Design review of the part built by this model. Coordinates are the model's own, in mm. A direction names the side the tool comes from. Coordinates: 2 decimals unless noted, no trailing zeros. Write each loop counter-clockwise with the first axis right and the second up, starting at its lowest first coordinate (ties: lowest second). Pieces come first, ordered by that corner, then holes. Notation, with made-up numbers: M 55.25,68.5 L 87.25,68.5 A16 cw 87.25,89.5 Z; hole C 39,32 d1. An arc over 180 degrees is marked long. Return JSON: item names as keys, results as strings. Group by question number.
```python
from build123d import *

# Parameters (mm, degrees)
CYLINDER001_R               = 4
CYLINDER001_DEPTH           = 30
CYLINDER_R                  = 2.2
CYLINDER_DEPTH              = 30
COMPOUND001_PLACEMENT_ANGLE = 60
BOX001_W                    = 114
BOX001_H                    = 52.5
BOX001_DEPTH                = 20
BOX002_W                    = 94
BOX002_H                    = 32.5
BOX002_DEPTH                = 20
BOX003_W                    = 74
BOX003_H                    = 10
BOX003_DEPTH                = 15
CYLINDER002_R               = 10
CYLINDER002_DEPTH           = 50
PAD_DEPTH                   = 4
PAD001_DEPTH                = 20
CYLINDER003_W               = 2.5
CYLINDER003_H               = 5
CYLINDER003_ANGLE           = 180
COMPOUND002_PLACEMENT_ANGLE = 60
BOX_W                       = 120
BOX_H                       = 58.5
BOX_DEPTH                   = 20
FILLET_R                    = 2


with BuildPart() as bolt_head_hole:
    # Cylinder001 → Cylinder001 (new body)
    with BuildSketch(Plane.XZ.offset(14)):
        Circle(CYLINDER001_R)
    extrude(amount=CYLINDER001_DEPTH)


with BuildPart() as bolt_hole_array_compound:
    # Cylinder → Cylinder (new body)
    with BuildSketch(Plane.XZ):
        Circle(CYLINDER_R)
    extrude(amount=CYLINDER_DEPTH)

    # Fusion002: union bolt head hole
    add(bolt_head_hole.part)


with BuildPart() as bolt_hole_array_compound_1:
    # Compound001 placement: moved
    add(bolt_hole_array_compound.part.moved(Location((-32.3149, 81.256849, 10))).rotate(Axis((-32.3149, 81.256849, 10), (0, 0, -1)), COMPOUND001_PLACEMENT_ANGLE))


with BuildPart() as part_mirroring:
    # Part__Mirroring: instance of bolt hole array compound
    add(bolt_hole_array_compound_1.part.mirror(Plane(origin=(0, 0, 0), x_dir=(0, -1, 0), z_dir=(1, 0, 0))))


with BuildPart() as obj1:
    # Box001 → Box001 (new body)
    with BuildSketch(Plane(origin=(-57, -26.25, 3), x_dir=(1, 0, 0), z_dir=(0, 0, 1))):
        with Locations((57, 26.25)):
            Rectangle(BOX001_W, BOX001_H)
    extrude(amount=BOX001_DEPTH)


with BuildPart() as obj2:
    # Box002 → Box002 (new body)
    with BuildSketch(Plane(origin=(-47, -16.25, 0), x_dir=(1, 0, 0), z_dir=(0, 0, 1))):
        with Locations((47, 16.25)):
            Rectangle(BOX002_W, BOX002_H)
    extrude(amount=BOX002_DEPTH)


with BuildPart() as switch_pocket:
    # Box003 → Box003 (new body)
    with BuildSketch(Plane(origin=(-37, -31.25, 8), x_dir=(1, 0, 0), z_dir=(0, 0, 1))):
        with Locations((37, 5)):
            Rectangle(BOX003_W, BOX003_H)
    extrude(amount=BOX003_DEPTH)


with BuildPart() as center_remove_cylinder:
    # Cylinder002 → Cylinder002 (new body)
    with BuildSketch(Plane(origin=(0, 47, -25), x_dir=(1, 0, 0), z_dir=(0, 0, 1))):
        Circle(CYLINDER002_R)
    extrude(amount=CYLINDER002_DEPTH)


with BuildPart() as extract_fusion:
    # Fusion003 base: copy of bolt hole array compound
    add(bolt_hole_array_compound_1.part)

    # Fusion003: union Part__Mirroring, obj1, obj2, switch pocket, center remove cylinder
    add(part_mirroring.part)
    add(obj1.part)
    add(obj2.part)
    add(switch_pocket.part)
    add(center_remove_cylinder.part)


with BuildPart() as bottom_body:
    # Sketch → Pad (new body)
    with BuildSketch(Plane.XY):
        with BuildLine():
            Line((-60, 29.25), (60, 29.25))
            Line((60, 29.25), (47.625, 86.066815))
            Line((32.625, 60.086053), (47.625, 86.066815))
            ThreePointArc((-32.625, 60.086053), (0, 41.25), (32.625, 60.086053))
            Line((-32.625, 60.086053), (-47.625, 86.066815))
            Line((-60, 29.25), (-47.625, 86.066815))
        make_face()
    extrude(amount=PAD_DEPTH)


with BuildPart() as bolt_wall_body:
    # Sketch001 → Pad001 (new body)
    with BuildSketch(Plane.XY):
        with BuildLine():
            Line((-47.625, 86.066815), (-32.625, 60.086053))
            ThreePointArc((-32.625, 60.086053), (0, 41.25), (32.625, 60.086053))
            Line((32.625, 60.086053), (47.625, 86.066815))
            Line((50.123562, 74.595272), (47.625, 86.066815))
            Line((44.094416, 64.152484), (50.123562, 74.595272))
            ThreePointArc((44.094416, 64.152484), (42.751879, 58.90179), (44.333925, 53.718226))
            Line((44.333925, 53.718226), (60, 29.25))
            Line((60, 29.25), (-60, 29.25))
            Line((-44.333925, 53.718226), (-60, 29.25))
            ThreePointArc((-44.333925, 53.718226), (-42.751879, 58.90179), (-44.094416, 64.152484))
            Line((-50.123562, 74.595272), (-44.094416, 64.152484))
            Line((-50.123562, 74.595272), (-47.625, 86.066815))
        make_face()
    extrude(amount=PAD001_DEPTH)


with BuildPart() as bolt_hole_array_compound001:
    # Cylinder003 → Cylinder003 (revolve)
    with BuildSketch(Plane(origin=(0, 0, 0), x_dir=(0, 0, -1), z_dir=(0, -1, 0))):
        with Locations((1.25, 2.5)):
            Rectangle(CYLINDER003_W, CYLINDER003_H)
    revolve(axis=Axis((0, 0, 0), (1, 0, 0)), revolution_arc=CYLINDER003_ANGLE)


with BuildPart() as bolt_hole_array_compound001_1:
    # Compound002 placement: moved
    add(bolt_hole_array_compound001.part.moved(Location((-39.21, 68.392051, 10))).rotate(Axis((-39.21, 68.392051, 10), (0, 0, -1)), COMPOUND002_PLACEMENT_ANGLE))


with BuildPart() as part_mirroring003:
    # Part__Mirroring003: instance of bolt hole array compound001
    add(bolt_hole_array_compound001_1.part.mirror(Plane(origin=(0, 0, 0), x_dir=(0, -1, 0), z_dir=(1, 0, 0))))


with BuildPart() as bolt_wall_body_cut:
    # Box → Box (new body)
    with BuildSketch(Plane(origin=(-60, -29.25, 0), x_dir=(1, 0, 0), z_dir=(0, 0, 1))):
        with Locations((60, 29.25)):
            Rectangle(BOX_W, BOX_H)
    extrude(amount=BOX_DEPTH)

    # Fillet
    fillet_edges = [bolt_wall_body_cut.edges().sort_by_distance(p)[0] for p in [
        (-60, -29.25, 10),
        (60, -29.25, 10),
    ]]
    fillet(fillet_edges, radius=FILLET_R)

    # Fusion: union bottom_body, bolt wall body, bolt hole array compound001, Part__Mirroring003
    add(bottom_body.part)
    add(bolt_wall_body.part)
    add(bolt_hole_array_compound001_1.part)
    add(part_mirroring003.part)

    # Cut001: cut extract fusion
    add(extract_fusion.part, mode=Mode.SUBTRACT)


solid = bolt_wall_body_cut.part
```
Item 1: The part is to be moulded in two halves that separate along X. For faces 4 (the flat face through (46.397, 68.14, 11.888)), 5 (the flat face through (40.02, 72.895, 9.86)), 6 (the flat face through (-0.8, -29.25, 7.6)), say which applies: pulls with the +X half, pulls with the -X half, needs draft (parallel to the pull), parting line crosses it, or undercut.
Item 2: Add section A-A (x = 0). Write out the cut boundary in (y, z), plus the area to 3 significant figures.
Item 3: For line 1 (X direction, y = -20, z = 17.5); line 2 (X direction, y = -9, z = 1); line 3 (Y direction, x = -4, z = 1.5), list the stretches that pass through material, from the lowest coordinate up.
Item 4: Add section D-D (z = 17.25). Write out the cut boundary in (x, y) (3 decimals), plus the area to 3 significant figures.
Item 5: Add section B-B (y = 10.5). Write out the cut boundary in (x, z), plus the area to 3 significant figures.
Item 6: Add section C-C (z = 1.5). Write out the cut boundary in (x, y) (3 decimals), plus the area to 3 significant figures.
Item 7: Machinability: for faces 1 (the flat face through (51, 52, 4)), 2 (the flat face through (57, 0, 11)), 3 (the flat face through (-1, -16.25, 1)), which of the approach directions +Z, -Z, +X, -X, +Y, -Y give a long, thin tool a straight path to every point of the face, cutting with its end or side? Answer none if there is none.
Item 8: For pin 1 (10 mm diameter, centred on x = -2, z = 18, fed in from -Y); pin 2 (0.9 mm diameter, centred on x = 8, y = -27.5, fed in from +Z); pin 3 (3.5 mm diameter, centred on x = 0, z = 1.5, fed in from +Y), all flat-tipped, find the tip position at first contact; note any pin that passes through.
Geometry check:
{
 "1": {"face 4": "pulls with the +X half", "face 5": "undercut", "face 6": "needs draft"},
 "2": {"outline": "M -29.25,0 L -16.25,0 L -16.25,3 L -26.25,3 L -26.25,8 L -29.25,8 Z; M 16.25,0 L 37,0 L 37,20 L 26.25,20 L 26.25,3 L 16.25,3 Z", "area": "299 mm^2"},
 "3": {"line 1": "-60 to -57, 57 to 60", "line 2": "-60 to -47, 47 to 60", "line 3": "-29.25 to -16.25, 16.25 to 37.83"},
 "4": {"outline": "M -60,-27.25 A2 ccw -58,-29.25 L -37,-29.25 L -37,-26.25 L -57,-26.25 L -57,26.25 L 57,26.25 L 57,-26.25 L 37,-26.25 L 37,-29.25 L 58,-29.25 A2 ccw 60,-27.25 L 60,29.25 L 44.334,53.718 A10.041 cw 44.094,64.152 L 50.124,74.595 L 47.625,86.067 L 32.625,60.086 A37.672 cw 8.826,42.298 A10 cw -8.826,42.298 A37.672 cw -32.625,60.086 L -47.625,86.067 L -50.124,74.595 L -44.094,64.152 A10.041 cw -44.334,53.718 L -60,29.25 Z", "area": "3,360 mm^2"},
 "5": {"outline": "M -60,0 L -47,0 L -47,3 L -57,3 L -57,20 L -60,20 Z; M 47,0 L 60,0 L 60,20 L 57,20 L 57,3 L 47,3 Z", "area": "180 mm^2"},
 "6": {"outline": "M -60,-27.25 A2 ccw -58,-29.25 L 58,-29.25 A2 ccw 60,-27.25 L 60,29.25 L 47.625,86.067 L 32.625,60.086 A37.672 cw 8.826,42.298 A10 cw -8.826,42.298 A37.672 cw -32.625,60.086 L -47.625,86.067 L -60,29.25 Z; hole M -47,-16.25 L 47,-16.25 L 47,16.25 L -47,16.25 Z", "area": "7,070 mm^2"},
 "7": {"face 1": "+Z, +X", "face 2": "+Z", "face 3": "+Z, -Z"},
 "8": {"pin 1": "y = 26.25", "pin 2": "z = 8", "pin 3": "y = 37.15"}
}
